Work out the finished part from the listing and answer in its coordinate system (mm). Face numbers are marked on the shaded views. A direction names the side the tool comes from. Coordinates: 2 decimals unless noted, no trailing zeros. Order: outer loops, then holes, each group sorted by start corner. A loop starts at its lowest first (then second) coordinate and runs counter-clockwise, first axis right, second up. Notation, with made-up numbers: M -6.5,-14.5 L 34.5,-14.5 A15 cw 34.5,-7.5 Z; hole C 19.5,-33.75 d4. An arc over 180 degrees is marked long. Use a Markdown table: item, result.
from build123d import *

# Parameters (mm, degrees)
BOSS_EXTRUDE1_DEPTH = 4.5
BOSS_EXTRUDE2_DEPTH = 3.8
BOSS_EXTRUDE3_DEPTH = 8.1


with BuildPart() as part:
    # Sketch1 → Boss-Extrude1 (new body)
    with BuildSketch(Plane(origin=(0, 0, 0), x_dir=(1, 0, 0), z_dir=(0, 1, 0))):
        with BuildLine():
            Line((7.25, 0), (7.25, -35))
            ThreePointArc((7.25, -35), (0, -42.25), (-7.25, -35))
            Line((-7.25, -35), (-7.25, 0))
            ThreePointArc((-7.25, 0), (0, 7.25), (7.25, 0))
        make_face()
    extrude(amount=BOSS_EXTRUDE1_DEPTH)

    # Sketch3 → Boss-Extrude2 (add)
    with BuildSketch(Plane(origin=(0, 4.5, 0), x_dir=(1, 0, 0), z_dir=(0, 1, 0))):
        with BuildLine():
            Line((-2.622571491, -0.457666807), (-2.622571491, -0.011296081))
            Line((-2.622571491, -0.011296081), (2.763792269, -0.011296081))
            Line((2.763792269, -0.011296081), (2.763792269, -0.457666807))
            ThreePointArc((2.763792269, -0.457666807), (2.791332039, -0.235236185), (2.800532634, -0.011296081))
            ThreePointArc((2.800532634, -0.011296081), (-0.153329714, 2.709425568), (-2.622571491, -0.457666807))
        make_face()
        with BuildLine():
            Line((2.763792269, -0.011296081), (-2.622571491, -0.011296081))
            Line((-2.622571491, -0.011296081), (-2.622571491, -0.457666807))
            ThreePointArc((-2.622571491, -0.457666807), (0.070610389, -2.741218326), (2.763792269, -0.457666807))
            Line((2.763792269, -0.457666807), (2.763792269, -0.011296081))
        make_face()
        with BuildLine():
            ThreePointArc((2.763792269, -0.457666807), (0.070610389, -2.741218326), (-2.622571491, -0.457666807))
            Line((-2.622571491, -0.457666807), (-2.622571491, -35.011296081))
            ThreePointArc((-2.622571491, -35.011296081), (0.070610389, -32.318114201), (2.763792269, -35.011296081))
            Line((2.763792269, -35.011296081), (2.763792269, -0.457666807))
        make_face()
        with BuildLine():
            ThreePointArc((2.763792269, -35.011296081), (0.070610389, -32.318114201), (-2.622571491, -35.011296081))
            Line((-2.622571491, -35.011296081), (2.763792269, -35.011296081))
        make_face()
        with BuildLine():
            Line((2.763792269, -35.011296081), (-2.622571491, -35.011296081))
            ThreePointArc((-2.622571491, -35.011296081), (0.070610389, -37.704477961), (2.763792269, -35.011296081))
        make_face()
    extrude(amount=BOSS_EXTRUDE2_DEPTH)

    # Sketch4 → Boss-Extrude3 (add)
    with BuildSketch(Plane(origin=(0, 8.3, 0), x_dir=(1, 0, 0), z_dir=(0, 1, 0))):
        with BuildLine():
            Line((7.25308141, 0.014627933), (7.323691799, -34.996668148))
            ThreePointArc((7.323691799, -34.996668148), (0.085238322, -42.264377491), (-7.182471021, -35.025924014))
            Line((-7.182471021, -35.025924014), (-7.25308141, -0.014627933))
            ThreePointArc((-7.25308141, -0.014627933), (-0.014627933, 7.25308141), (7.25308141, 0.014627933))
        make_face()
    extrude(amount=BOSS_EXTRUDE3_DEPTH)


solid = part.part
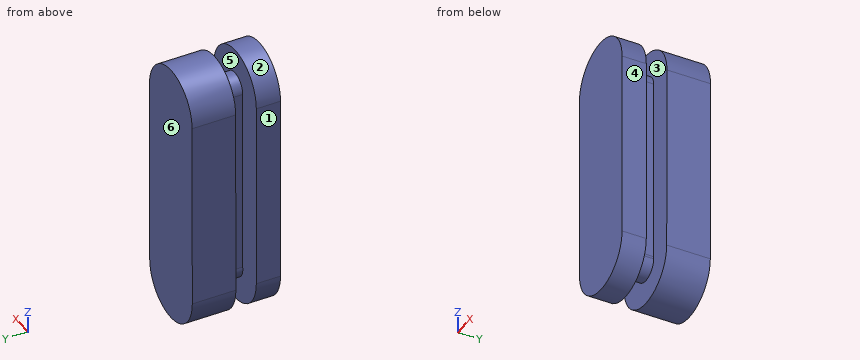
(1) A cutting plane is placed at C-C (x = 0). Determine the outline of the cut face in (y, z).
Conclusion:
| item | result |
|---|---|
| outline | M 0,-7.25 L 4.5,-7.25 L 4.5,-2.72 L 8.3,-2.72 L 8.3,-7.25 L 16.4,-7.25 L 16.4,42.26 L 8.3,42.26 L 8.3,37.7 L 4.5,37.7 L 4.5,42.25 L 0,42.25 Z |
(2) Straight lines are drawn through the part: L1, parallel to Y at x = -5.75, z = 38; L2, parallel to X at y = 10, z = 3; L3, parallel to X at y = 6.5, z = 4. For each, find the intervals that lie inside material, in ascending order.
Conclusion:
| item | result |
|---|---|
| L1 | 0 to 4.5, 8.3 to 16.4 |
| L2 | -7.25 to 7.26 |
| L3 | -2.62 to 2.76 |
(3) Determine the mould class of the marked faces 3, 4, 5 and 6 for opening direction Y: pulls with the +Y half, pulls with the -Y half, needs draft (parallel to the pull), parting line crosses it, or undercut.
Conclusion:
| item | result |
|---|---|
| face 3 | undercut |
| face 4 | needs draft |
| face 5 | undercut |
| face 6 | pulls with the +Y half |
(4) A cutting plane is placed at A-A (x = -5.5). Determine the outline of the cut face in (y, z), then the cut area to 3 significant figures.
Conclusion:
| item | result |
|---|---|
| outline | M 0,-4.72 L 4.5,-4.72 L 4.5,39.72 L 0,39.72 Z; M 8.3,-4.73 L 16.4,-4.73 L 16.4,39.66 L 8.3,39.66 Z |
| area | 560 mm2 |
(5) Given P1, Ø6, axis at y = 12, z = 8, coming from the -X side; P2, Ø1.1, axis at y = 7, z = 26.5, coming from the +X side; P3, Ø5, axis at y = 1.5, z = 25, coming from the +X side, each flat-ended and moving along its own axis, determine where each tip first touches the part or whether it passes through.
Conclusion:
| item | result |
|---|---|
| P1 | x = -7.24 |
| P2 | x = 2.76 |
| P3 | x = 7.25 |
(6) Which of the six approach directions +Z, -Z, +X, -X, +Y, -Y give full straight-line access (tool end or side, diameter ignored) to the marked faces 1 and 2?
Conclusion:
| item | result |
|---|---|
| face 1 | +Z, -Z, -X, +Y, -Y |
| face 2 | +Z, -Y |
(7) A cutting plane is placed at B-B (z = 37). Determine the outline of the cut face in (x, y), then the cut area to 3 significant figures.
Conclusion:
| item | result |
|---|---|
| outline | M -6.97,0 L 6.97,0 L 6.97,4.5 L 1.89,4.5 L 1.89,8.3 L 7.05,8.3 L 7.05,16.4 L -6.9,16.4 L -6.9,8.3 L -1.75,8.3 L -1.75,4.5 L -6.97,4.5 Z |
| area | 190 mm2 |
(8) A cutting plane is placed at D-D (y = 7). Determine the outline of the cut face in (x, z), then the cut area to 3 significant figures.
Conclusion:
| item | result |
|---|---|
| outline | M -2.62,0.46 A2.73 ccw long 2.76,0.46 L 2.76,35.01 A2.69 ccw -2.62,35.01 Z |
| area | 212 mm2 |
